from build123d import *

# Parameters (mm, degrees)
F0_R     = 12.7
F1_DEPTH = 76.2


with BuildPart() as f1:
    # F0 (on Top) → F1 (new body)
    with BuildSketch(Plane.XY):
        Circle(F0_R)
    extrude(amount=F1_DEPTH)

    # F2 (on Front) → F3 (revolve)
    with BuildSketch(Plane.XZ):
        with BuildLine():
            ThreePointArc((0, 57.15), (19.05, 76.2), (0, 95.25))
            Line((0, 95.25), (0, 76.2))
            Line((0, 76.2), (0, 57.15))
        make_face()
    revolve(axis=Axis((0, 0, 85.725), (0, 0, -1)))

    # F4 (on Front) → F5 (revolve)
    with BuildSketch(Plane.XZ):
        with BuildLine():
            Line((0, 0), (0, -19.05))
            ThreePointArc((0, -19.05), (19.05, 0), (0, 19.05))
            Line((0, 19.05), (0, 0))
        make_face()
    revolve(axis=Axis((0, 0, -9.525), (0, 0, 1)))


solid = f1.part
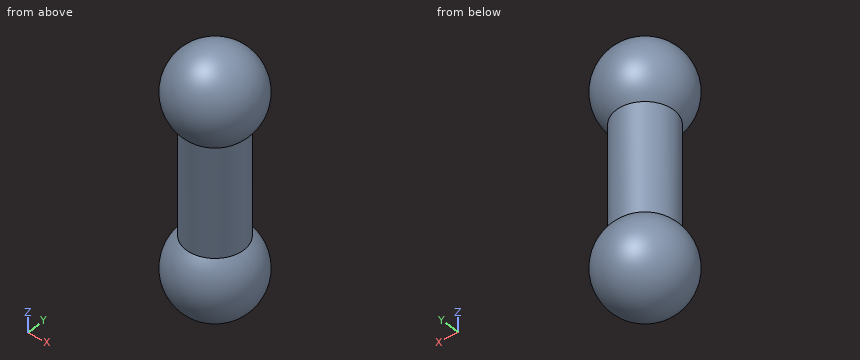
Verification items for the finished model (mm, model axes). Give positions to 0.01 mm unless a question says otherwise; leave off trailing zeros. Loops run counter-clockwise (first coordinate to the right, second up) from the corner with the lowest first, then second, coordinate; pieces in that order, holes last.
1) Thickness scan on line 1 along Z through (x, y) = (-7.5, -13.5); line 2 along Z through (x, y) = (12, 13); line 3 along X through (y, z) = (-10.5, 87.5). Record the ranges inside material, lowest first.
2) Sectioned sample at C-C, the plane z = -6.5. Enter the section's corners in (x, y), then the cut area to 3 significant figures.
3) Sectioned sample at A-A, the plane x = 0. Enter the section's corners in (y, z).
4) Sectioned sample at D-D, the plane z = 13. Enter the section's corners in (x, y).
5) Depth check by flat-ended pin: pin 1 Ø12 at (x, z) = (14.5, 15) entering from -Y; pin 2 Ø1 at (y, z) = (-7, 13.5) entering from -X; pin 3 Ø8 at (y, z) = (-11.5, 0) entering from -X. Enter the tip coordinate at first touch or a pass-through.
Answers:
1. line 1: z = -11.15 to 11.15, 65.05 to 87.35
1. line 2: z = -7.06 to 7.06, 69.14 to 83.26
1. line 3: x = -11.18 to 11.18
2. outline: circle Ø35.81 at (0, 0)
2. area: 1,010 mm2
3. outline: (-12.7, 14.2) arc R19.05 ccw (long way) to (12.7, 14.2) - (12.7, 62) arc R19.05 ccw (long way) to (-12.7, 62) - close
4. outline: circle Ø27.85 at (0, 0)
5. pin 1: stops at y = -11.92
5. pin 2: stops at x = -12.11
5. pin 3: stops at x = -17.51
